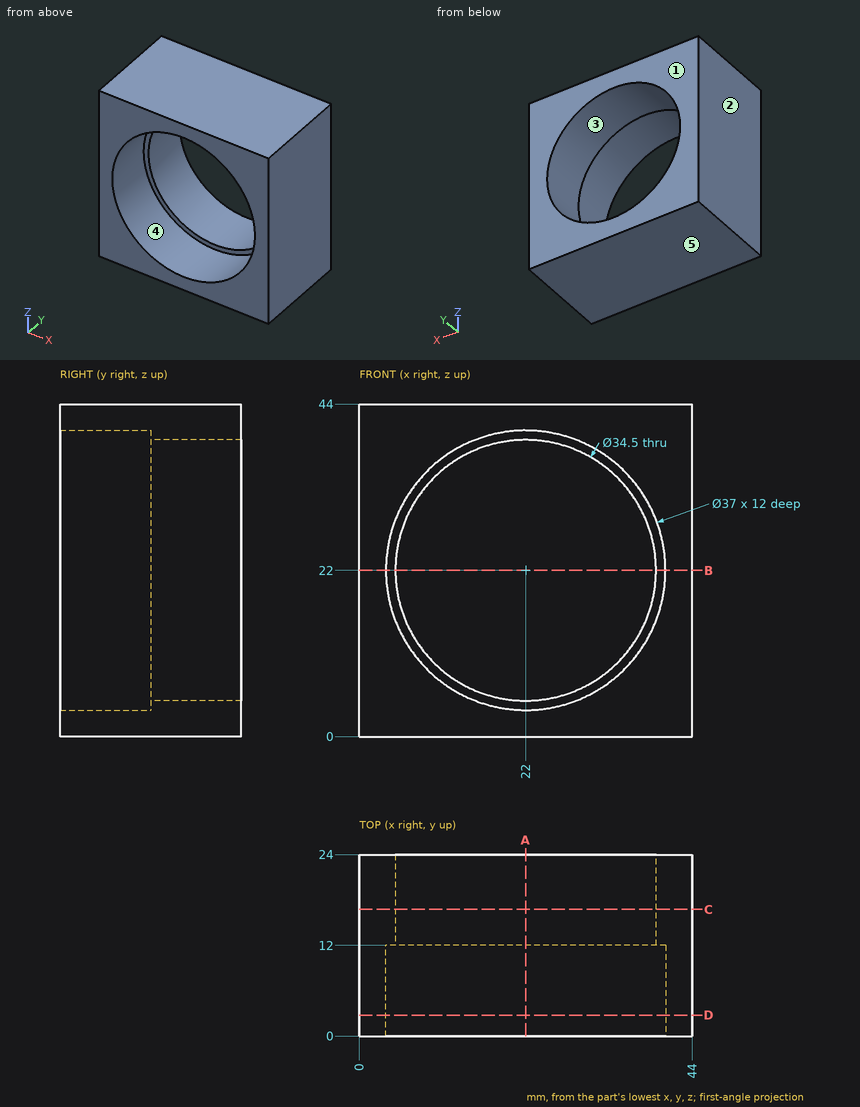
Study the drawing (mm; zero at the part's minimum x, y, z) and answer. A direction names the side the tool comes from. Give positions to 0.01 mm unless a question says otherwise; leave off trailing zeros. Write each loop counter-clockwise with the first axis right and the second up, starting at its lowest first coordinate (ties: lowest second). Pieces come first, ordered by that corner, then holes.
Item 1: Determine the mould class of the marked faces 1, 2 and 3 for opening direction X: released by +X, released by -X, zero draft, split by the parting line, or undercut.
Item 2: Find the intervals of material crossed by line 1 along Z through (x, y) = (22, 4); line 2 along Z through (x, y) = (22, 17); line 3 along X through (y, z) = (14.5, 22.5), in increasing order.
Item 3: Section C-C, the plane y = 16.75 is taken. Write down the section's boundary in (x, z).
Item 4: Section A-A, the plane x = 22 is taken. Write down the section's boundary in (y, z), plus the area to 3 significant figures.
Item 5: Section D-D, the plane y = 2.75 is taken. Write down the section's boundary in (x, z).
Item 6: Which of the six approach directions +Z, -Z, +X, -X, +Y, -Y give full straight-line access (tool end or side, diameter ignored) to the marked faces 4 and 5?
Item 7: Section B-B, the plane z = 22 is taken. Write down the section's boundary in (x, y).
Completed:
1. face 1: zero draft
1. face 2: released by -X
1. face 3: undercut
2. line 1: z = 0 to 3.5, 40.5 to 44
2. line 2: z = 0 to 4.75, 39.25 to 44
2. line 3: x = 0 to 4.76, 39.24 to 44
3. outline: (0, 0) - (44, 0) - (44, 44) - (0, 44) - close; hole circle Ø34.5 at (22, 22)
4. outline: (0, 0) - (24, 0) - (24, 4.75) - (12, 4.75) - (12, 3.5) - (0, 3.5) - close; (0, 40.5) - (12, 40.5) - (12, 39.25) - (24, 39.25) - (24, 44) - (0, 44) - close
4. area: 198 mm2
5. outline: (0, 0) - (44, 0) - (44, 44) - (0, 44) - close; hole circle Ø37 at (22, 22)
6. face 4: -Y
6. face 5: -Z, +X, -X, +Y, -Y
7. outline: (0, 0) - (3.5, 0) - (3.5, 12) - (4.75, 12) - (4.75, 24) - (0, 24) - close; (39.25, 12) - (40.5, 12) - (40.5, 0) - (44, 0) - (44, 24) - (39.25, 24) - close
